from build123d import *

# Parameters (mm, degrees)
SKETCH_1_R          = 6
EXTRUDE_1_DEPTH     = 8
EXTRUDE_1_2_DEPTH   = 8
EXTRUDE_1_3_DEPTH   = 8
SKETCH_3_R          = 2.5
CUT_EXTRUDE_1_DEPTH = 9
SKETCH_4_R          = 2
CUT_EXTRUDE_2_DEPTH = 9
SKETCH_5_R          = 4
CUT_EXTRUDE_3_DEPTH = 4.5
CHAMFER_1_SIZE      = 0.3


with BuildPart() as part:
    # 草图1 → Extrude 1 (new body)
    with BuildSketch(Plane.XY):
        Circle(SKETCH_1_R)
    extrude(amount=EXTRUDE_1_DEPTH)



with BuildPart() as body_2:
    # 草图1 → Extrude 1 2 (new body)
    with BuildSketch(Plane.XY):
        with Locations((0, 135)):
            Circle(SKETCH_1_R)
    extrude(amount=EXTRUDE_1_2_DEPTH)


with BuildPart() as part_1:
    add(part.part)

    add(body_2.part)  # Extrude 1 3 merges body 2
    # 草图2 → Extrude 1 3 (add)
    with BuildSketch(Plane.XY):
        with BuildLine():
            Line((-4.330127019, 132.5), (4.330127019, 117.5))
            ThreePointArc((4.330127019, 117.5), (4.829629131, 116.294095226), (5, 115))
            Line((5, 115), (5, 20))
            ThreePointArc((5, 20), (4.829629131, 18.705904774), (4.330127019, 17.5))
            Line((4.330127019, 17.5), (-4.330127019, 2.5))
            Line((-4.330127019, 2.5), (4.330127019, -2.5))
            Line((4.330127019, -2.5), (12.990381057, 12.5))
            ThreePointArc((12.990381057, 12.5), (14.488887394, 16.117714323), (15, 20))
            Line((15, 20), (15, 115))
            ThreePointArc((15, 115), (14.488887394, 118.882285677), (12.990381057, 122.5))
            Line((12.990381057, 122.5), (4.330127019, 137.5))
            Line((4.330127019, 137.5), (-4.330127019, 132.5))
        make_face()
    extrude(amount=EXTRUDE_1_3_DEPTH)

    # 草图3 → 切除-拉伸1 (cut, through all)
    with BuildSketch(Plane.XY.offset(8)):
        Circle(SKETCH_3_R)
    extrude(amount=-CUT_EXTRUDE_1_DEPTH, mode=Mode.SUBTRACT)

    # 草图4 → 切除-拉伸2 (cut, through all)
    with BuildSketch(Plane(origin=(0, 0, 0), x_dir=(-1, 0, 0), z_dir=(0, 0, -1))):
        with Locations((0, 135)):
            Circle(SKETCH_4_R)
    extrude(amount=-CUT_EXTRUDE_2_DEPTH, mode=Mode.SUBTRACT)

    # 草图5 → 切除-拉伸3 (cut)
    with BuildSketch(Plane(origin=(0, 0, 0), x_dir=(-1, 0, 0), z_dir=(0, 0, -1))):
        with Locations((0, 135)):
            Circle(SKETCH_5_R)
    extrude(amount=-CUT_EXTRUDE_3_DEPTH, mode=Mode.SUBTRACT)

    # 倒角1
    chamfer_1_edges = [part_1.edges().sort_by_distance(p)[0] for p in [
        (0.829156198, 11.436140662, 0),
        (9.489410235, 6.436140662, 8),
        (14.488887394, 16.117714323, 8),
        (15, 67.5, 8),
        (14.488887394, 118.882285677, 8),
        (4.829629131, 116.294095226, 0),
        (5, 67.5, 0),
        (4.829629131, 18.705904774, 0),
        (9.489410235, 6.436140662, 0),
        (14.488887394, 118.882285677, 0),
        (15, 67.5, 0),
        (14.488887394, 16.117714323, 0),
        (4.829629131, 116.294095226, 8),
        (5, 67.5, 8),
        (4.829629131, 18.705904774, 8),
        (0.829156198, 11.436140662, 8),
        (0.829156198, 123.563859338, 8),
        (0.829156198, 123.563859338, 0),
        (9.489410235, 128.563859338, 8),
        (9.489410235, 128.563859338, 0),
        (-3, 140.196152423, 0),
        (-3, 140.196152423, 8),
        (-2.5, 0, 0),
        (-2.5, 0, 8),
        (-3, -5.196152423, 0),
        (2, 135, 8),
        (4, 135, 0),
        (-3, -5.196152423, 8),
    ]]
    chamfer(chamfer_1_edges, length=CHAMFER_1_SIZE)


solid = part_1.part
Check sheet for the modelled part. Datum: model origin and axes. Units: mm. A direction names the side the tool comes from. Round coordinates to 2 decimals unless told otherwise and drop trailing zeros. Loops run counter-clockwise (first coordinate to the right, second up) from the corner with the lowest first, then second, coordinate; pieces in that order, holes last. Notation, with made-up numbers: (-21, -6) - (-6, -6) arc R29 ccw to (-6, 24) - close; hole circle Ø10 at (68, 32). An arc over 180 degrees is marked (long way). Answer as CSV lines item,"result". Start each with the question number.
Item 1: Set-up check for faces 1 (the flat face through (0.78, 123.65, 3.95)), 2 (the flat face through (-1, 137, 4.5)), 3 (the flat face through (9.29, 6.39, 7.85)), 4 (the flat face through (0.889, 123.765, 7.852)): record each of +Z, -Z, +X, -X, +Y, -Y from which the full face is reachable in a straight line by a thin tool's end or side.
Item 2: Depth check by flat-ended pin: P1, Ø1, axis at y = 31, z = 6, coming from the -X side; P2, Ø2.5, axis at x = -1.5, y = 136, coming from the -Z side; P3, Ø2.5, axis at x = 0, y = 135, coming from the -Z side. Enter the tip coordinate at first touch or a pass-through.
Item 3: Scan lines: line 1 (X direction, y = 135, z = 5.85); line 2 (Y direction, x = 0, z = 3.05); line 3 (Y direction, x = 0, z = 5.25). Record each from-to range of solid material in increasing order. Write a range as [from, to].
Item 4: Section check C-C (x = 11.5). Record the boundary of the cut face in (y, z).
Item 5: Section check D-D (x = 0). Count the separate pieces of the cut face and the enclosed holes in it, and give its area (3 significant figures).
Item 6: Section check B-B (z = 3.25). Record the boundary of the cut face in (x, y).
Item 7: Release check for a two-part mould opening along Y. For faces 5 (the conical face through (14.3, 16.11, 0.12)), 6 (the conical face through (-2.75, -5.13, 0.12)), 7 (the flat face through (0.99, 11.41, 7.85)), 8 (the cylindrical face through (14.503, 118.829, 3.948)) record: +Y half, -Y half, draft (parallel to the pull), parting line (faces both ways), or undercut.
Item 8: Section check A-A (y = 86.5). Record the boundary of the cut face in (x, z), and give its area (3 significant figures).
Report:
1,face 1,"+Z, -Z, -X"
1,face 2,"-Z"
1,face 3,"+Z, +X, -Y"
1,face 4,"+Z, -X"
2,P1,"stops at x = 5"
2,P2,"stops at z = 4.5"
2,P3,"passes through"
3,line 1,"x = [-6, -2], [2, 6]"
3,line 2,"y = [-6, -2.5], [2.5, 10], [125, 131], [139, 141]"
3,line 3,"y = [-6, -2.5], [2.5, 10], [125, 133], [137, 141]"
4,outline,"(9.92, 0.3) - (10.52, 0) - (124.48, 0) - (125.08, 0.3) - (125.08, 7.7) - (124.48, 8) - (10.52, 8) - (9.92, 7.7) - close"
5,separate pieces,"4"
5,enclosed holes,"0"
5,area,"165 mm2"
6,outline,"(-2.67, 5.37) arc R6 ccw (long way) to (5.99, 0.37) - (12.99, 12.5) arc R15 ccw to (15, 20) - (15, 115) arc R15 ccw to (12.99, 122.5) - (5.99, 134.63) arc R6 ccw (long way) to (-2.67, 129.63) - (4.33, 117.5) arc R5 cw to (5, 115) - (5, 20) arc R5 cw to (4.33, 17.5) - close; hole circle Ø8 at (0, 135); hole circle Ø5 at (0, 0)"
7,face 5,"-Y half"
7,face 6,"undercut"
7,face 7,"undercut"
7,face 8,"+Y half"
8,outline,"(5, 0.3) - (5.3, 0) - (14.7, 0) - (15, 0.3) - (15, 7.7) - (14.7, 8) - (5.3, 8) - (5, 7.7) - close"
8,area,"79.8 mm2"
